Solid Edge part; units mm, degrees
sketch "Sketch1" plane through (0, 0, 0) normal (1, 0, 0) x (0, 1, 0)
  line L0 (27.5, -27) -> (27.5, 23)
  line L1 (27.5, 23) -> (-31.5, 23)
  line L2 (-31.5, 23) -> (-31.5, -27)
  line L3 (-31.5, -27) -> (27.5, -27)
extrude "Protrusion1" add sketch "Sketch1" along normal blind 2
sketch "Sketch2" plane through (0, 0, 0) normal (1, 0, 0) x (0, 1, 0)
  line L0 (-31.5, 21) -> (-7, 21)
  line L1 (-7, 21) -> (-7, 23)
  line L2 (-7, 23) -> (-31.5, 23)
  line L3 (-31.5, 23) -> (-31.5, 21)
extrude "ExtrudedCutout_1" cut sketch "Sketch2" along normal blind 2
sketch "Sketch3" plane through (0, 0, 0) normal (1, 0, 0) x (0, 1, 0)
  line L0 (3, 21) -> (27.5, 21)
  line L1 (27.5, 21) -> (27.5, 23)
  line L2 (27.5, 23) -> (3, 23)
  line L3 (3, 23) -> (3, 21)
extrude "ExtrudedCutout_2" cut sketch "Sketch3" along normal blind 2
sketch "Sketch4" plane through (0, 0, 0) normal (1, 0, 0) x (0, 1, 0)
  line L0 (23.5, 3) -> (23.5, -7)
  line L1 (23.5, -7) -> (25.5, -7)
  line L2 (25.5, -7) -> (25.5, 3)
  line L3 (25.5, 3) -> (23.5, 3)
extrude "ExtrudedCutout_3" cut sketch "Sketch4" along normal blind 2
sketch "Sketch5" plane through (0, 0, 0) normal (1, 0, 0) x (0, 1, 0)
  line L0 (27.5, -25) -> (3, -25)
  line L1 (3, -25) -> (3, -27)
  line L2 (3, -27) -> (27.5, -27)
  line L3 (27.5, -27) -> (27.5, -25)
extrude "ExtrudedCutout_4" cut sketch "Sketch5" along normal blind 4
sketch "Sketch6" plane through (0, 0, 0) normal (1, 0, 0) x (0, 1, 0)
  line L0 (-7, -25) -> (-31.5, -25)
  line L1 (-31.5, -25) -> (-31.5, -27)
  line L2 (-31.5, -27) -> (-7, -27)
  line L3 (-7, -27) -> (-7, -25)
extrude "ExtrudedCutout_5" cut sketch "Sketch6" along normal blind 2
sketch "Sketch7" plane through (0, 0, 0) normal (1, 0, 0) x (0, 1, 0)
  line L0 (-29.5, -7) -> (-27.5, -7)
  line L1 (-27.5, -7) -> (-27.5, 3)
  line L2 (-27.5, 3) -> (-29.5, 3)
  line L3 (-29.5, 3) -> (-29.5, -7)
extrude "ExtrudedCutout_6" cut sketch "Sketch7" along normal blind 4
sketch "Sketch8" plane through (0, 0, 0) normal (1, 0, 0) x (0, 1, 0)
  circle A0 centre (-11.5, 10) radius 1.6
  circle A1 centre (7.5, -14) radius 1.6
extrude "ExtrudedCutout_7" cut sketch "Sketch8" along normal blind 2
properties material "Acrylic, high impact grade"
Could you check a few things on this model? Use its own coordinates, in mm. A direction names the side the tool comes from. Give positions to 0.01 mm unless a question says otherwise; leave off trailing zeros. Order: outer loops, then holes, each group sorted by start corner. A loop starts at its lowest first (then second) coordinate and runs counter-clockwise, first axis right, second up.
1. We'd pull the mould along Z, two halves only. Please class faces 5 (the flat face through (1, 24, -7)), 6 (the flat face through (1, 27.5, -2)), 7 (the flat face through (1, -2, 23)): pulls with the +Z half, pulls with the -Z half, needs draft (parallel to the pull), parting line crosses it, or undercut.
2. Suppose I cut it at B-B (z = -1). List the corners of the cut face in (x, y) for me, plus the area to 3 significant figures.
3. For faces 1 (the flat face through (1, 23.5, -2)), 2 (the flat face through (1, 3, 22)), 3 (the flat face through (1, -7, 22)), 4 (the flat face through (1, -7, -26)), which set-ups out of +Z, -Z, +X, -X, +Y, -Y let a thin tool reach every point of the face, with its end or its side?
4. Suppose I cut it at C-C (z = -14). List the corners of the cut face in (x, y) for me.
5. Will these pins go through, and if not, where does the flat tip stop? P1, Ø3, axis at y = -11.5, z = 10, coming from the -X side; P2, Ø1, axis at x = 1, y = -28.5, coming from the -Z side; P3, Ø1, axis at x = 1.5, y = 8.5, coming from the +Z side.
6. I need wall thicknesses on L1, parallel to Y at x = 0.7, z = 0; L2, parallel to Z at x = 1.65, y = 7.5; L3, parallel to Z at x = 0.75, y = -11.5. Which ranges of each line are inside material? Lowest first, please.
7. Suppose I cut it at A-A (y = 7.5). List the corners of the cut face in (x, z) for me, plus the area to 3 significant figures.
8. Suppose I cut it at D-D (x = 0.45). List the corners of the cut face in (y, z) for me, plus the area to 3 significant figures.
Solved:
1. face 5: undercut
1. face 6: needs draft
1. face 7: pulls with the +Z half
2. outline: (0, -31.5) - (2, -31.5) - (2, -29.5) - (0, -29.5) - close; (0, -27.5) - (2, -27.5) - (2, 23.5) - (0, 23.5) - close; (0, 25.5) - (2, 25.5) - (2, 27.5) - (0, 27.5) - close
2. area: 110 mm2
3. face 1: +X, -X
3. face 2: +Z, +X, -X, +Y
3. face 3: +Z, +X, -X, -Y
3. face 4: -Z, +X, -X, -Y
4. outline: (0, -31.5) - (2, -31.5) - (2, 5.9) - (0, 5.9) - close; (0, 9.1) - (2, 9.1) - (2, 27.5) - (0, 27.5) - close
5. P1: passes through
5. P2: stops at z = -25
5. P3: stops at z = 21
6. L1: y = -31.5 to -29.5, -27.5 to 23.5, 25.5 to 27.5
6. L2: z = -25 to -15.6, -12.4 to 21
6. L3: z = -25 to 8.4, 11.6 to 21
7. outline: (0, -25) - (2, -25) - (2, -15.6) - (0, -15.6) - close; (0, -12.4) - (2, -12.4) - (2, 21) - (0, 21) - close
7. area: 85.6 mm2
8. outline: (-31.5, -25) - (-7, -25) - (-7, -27) - (3, -27) - (3, -25) - (27.5, -25) - (27.5, 21) - (3, 21) - (3, 23) - (-7, 23) - (-7, 21) - (-31.5, 21) - close; hole (-29.5, -7) - (-27.5, -7) - (-27.5, 3) - (-29.5, 3) - close; hole circle Ø3.2 at (-11.5, 10); hole circle Ø3.2 at (7.5, -14); hole (23.5, -7) - (25.5, -7) - (25.5, 3) - (23.5, 3) - close
8. area: 2,700 mm2
